Build history of the part. All positions in model axes, mm. Face numbers are marked on the shaded views. Round coordinates to 2 decimals unless told otherwise and drop trailing zeros. Loops run counter-clockwise (first coordinate to the right, second up) from the corner with the lowest first, then second, coordinate; pieces in that order, holes last. Notation, with made-up numbers: (37.25, -16) - (70.25, -16) arc R14 ccw to (70.25, 4) - close; hole circle Ø9 at (81.5, -14). An arc over 180 degrees is marked (long way). Put each result on its own line as item: value. Start each with the question number.
from build123d import *

# Parameters (mm, degrees)
SKETCH_W            = 310
SKETCH_H            = 360
PAD_DEPTH           = 27.5
SKETCH001_W         = 35
SKETCH001_H         = 35
PAD001_DEPTH        = 760
LINEARPATTERN_COUNT = 2
LINEARPATTERN_PITCH = 380
SKETCH002_W         = 31
SKETCH002_H         = 31
POCKET_DEPTH        = 28
SKETCH003_W         = 50
SKETCH003_H         = 50
POCKET001_DEPTH     = 5


with BuildPart() as part:
    # Sketch → Pad (new body)
    with BuildSketch(Plane.XY):
        Rectangle(SKETCH_W, SKETCH_H)
    pad = extrude(amount=PAD_DEPTH)

    # Sketch001 (on Face5 of Pad) → Pad001 (join)
    with BuildSketch(Plane(origin=(0, 0, 0), x_dir=(1, 0, 0), z_dir=(0, 0, -1))):
        with Locations((-137.5, 162.5)):
            Rectangle(SKETCH001_W, SKETCH001_H)
        with Locations((-137.5, -162.5)):
            Rectangle(SKETCH001_W, SKETCH001_H)
        with Locations((137.5, 162.5)):
            Rectangle(SKETCH001_W, SKETCH001_H)
        with Locations((137.5, -162.5)):
            Rectangle(SKETCH001_W, SKETCH001_H)
    extrude(amount=PAD001_DEPTH)

    # LinearPattern: Pad ×2
    with Locations(*[(0, 0, -i * LINEARPATTERN_PITCH) for i in range(1, LINEARPATTERN_COUNT)]):
        add(pad)

    # Sketch002 (on Face15 of LinearPattern) → Pocket (cut)
    with BuildSketch(Plane.XY.offset(27.5)):
        Rectangle(SKETCH002_W, SKETCH002_H)
    extrude(amount=-POCKET_DEPTH, mode=Mode.SUBTRACT)

    # Sketch003 (on Face16 of Pocket) → Pocket001 (cut)
    with BuildSketch(Plane.XY.offset(27.5)):
        Rectangle(SKETCH003_W, SKETCH003_H)
    extrude(amount=-POCKET001_DEPTH, mode=Mode.SUBTRACT)


solid = part.part
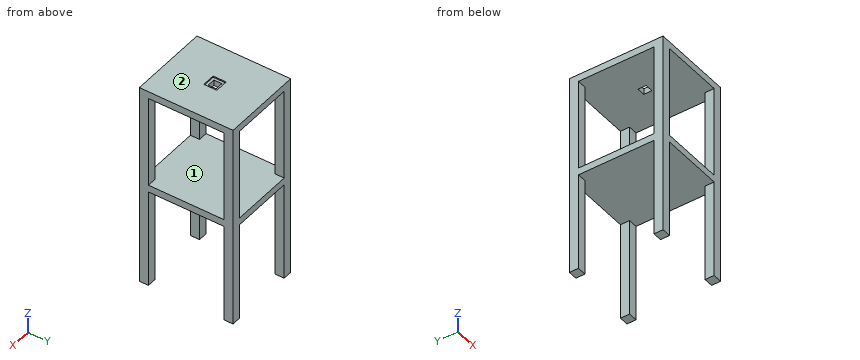
1) Slice it at A-A, the plane x = 111. Write the cut outline in (y, z).
2) Slice it at B-B, the plane z = -471. Write the cut outline in (x, y).
3) Slice it at C-C, the plane y = -129. Write the cut outline in (x, z), and give its area (4 significant figures).
4) Drill centre lines: line 1 (X direction, y = 165, z = -42); line 2 (Z direction, x = 11, y = -131); line 3 (Y direction, x = -127, z = -582.5). Where is each one in solid material? Low to high. Write a range as [from, to].
5) Drop a flat-ended pin along its axis: pin 1 Ø5 at (x, y) = (-76, -119) entering from -Z. Give the stop position or say it passes through.
6) Pull direction Z, two halves, no side cores. Call the marked faces 1 and 2: pulls with the +Z half, pulls with the -Z half, needs draft (parallel to the pull), parting line crosses it, or undercut.
Taken from the geometry:
1. outline: (-180, -380) - (180, -380) - (180, -352.5) - (-180, -352.5) - close; (-180, 0) - (180, 0) - (180, 27.5) - (-180, 27.5) - close
2. outline: (-155, -180) - (-120, -180) - (-120, -145) - (-155, -145) - close; (-155, 145) - (-120, 145) - (-120, 180) - (-155, 180) - close; (120, -180) - (155, -180) - (155, -145) - (120, -145) - close; (120, 145) - (155, 145) - (155, 180) - (120, 180) - close
3. outline: (-155, -380) - (155, -380) - (155, -352.5) - (-155, -352.5) - close; (-155, 0) - (155, 0) - (155, 27.5) - (-155, 27.5) - close
3. area: 17,050 mm2
4. line 1: x = [-155, -120], [120, 155]
4. line 2: z = [-380, -352.5], [0, 27.5]
4. line 3: y = [-180, -145], [145, 180]
5. pin 1: stops at z = -380
6. face 1: undercut
6. face 2: pulls with the +Z half
